Source: CAD feature listing. Evaluate the final solid. Frame: model axes, mm. A direction names the side the tool comes from. Round coordinates to 2 decimals unless told otherwise and drop trailing zeros. Order: outer loops, then holes, each group sorted by start corner. A loop starts at its lowest first (then second) coordinate and runs counter-clockwise, first axis right, second up. Notation, with made-up numbers: (59, 77) - (95, 77) arc R26 ccw to (95, 108) - close; hole circle Ø4 at (-4.5, 69). An arc over 180 degrees is marked (long way). Put each result on its own line as item: value. Start each with the question number.
1) Mould query, pull axis Z, two halves, no side actions, for faces 4 (the face through (-13, 16, 70)), 5 (the face through (3, 0, 100)), 6 (the face through (0, -2, 0)), 7 (the face through (-5, 5, 80)). Classes: +Z half, -Z half, draft (parallel to the pull), parting line (faces both ways), or undercut.
2) Access query for faces 1 (the face through (-13, 16, 50)), 2 (the face through (-14.985, 0.66, 23.269)), 3 (the face through (-1, 0, 115)). Directions: +Z, -Z, +X, -X, +Y, -Y. A direction counts if a zero-diameter tool reaches every point of the face in a straight line with its end or side. Return the directions, or none.
3) Line query: probe 1 along Z at (x, y) = (13, -17.5); probe 2 along Z at (x, y) = (5, 2); probe 3 along Z at (x, y) = (-9, -13.5). Output: solid intervals per line, ascending. Write a range as [from, to].
4) Section B-B on y = -17. Output: boundary loops of the cut face in (x, z), then the cut area to 3 significant figures.
5) Contact query for flat-ended pins moving along their axis: P1, Ø2, axis at y = 5.5, z = 19, coming from the -X side; P2, Ø0.6, axis at x = 4, y = 1, coming from the +Z side; P3, Ø4, axis at x = 7.5, y = -1, coming from the -Z side. Output: stop coordinate, or through.
6) Section A-A on z = 57. Output: boundary loops of the cut face in (x, y).
```python
from build123d import *

# Parameters (mm, degrees)
SKETCH1_R           = 15
BOSS_EXTRUDE1_DEPTH = 40
SKETCH2_W           = 42
SKETCH2_H           = 42
BOSS_EXTRUDE4_DEPTH = 10
SKETCH3_R           = 20
BOSS_EXTRUDE5_DEPTH = 20
SKETCH4_W           = 42
SKETCH4_H           = 42
BOSS_EXTRUDE6_DEPTH = 10
SKETCH5_R           = 5
BOSS_EXTRUDE7_DEPTH = 35
FILLET3_R           = 7
SKETCH6_R           = 1.25
BOSS_EXTRUDE8_DEPTH = 5
FILLET5_R           = 0.3
SKETCH7_W           = 4
SKETCH7_H           = 6
CUT_EXTRUDE1_DEPTH  = 30


with BuildPart() as part:
    # Sketch1 → Boss-Extrude1 (new body)
    with BuildSketch(Plane.XY):
        Circle(SKETCH1_R)
    extrude(amount=BOSS_EXTRUDE1_DEPTH)

    # Sketch2 → Boss-Extrude4 (add)
    with BuildSketch(Plane.XY.offset(40)):
        Rectangle(SKETCH2_W, SKETCH2_H)
    extrude(amount=BOSS_EXTRUDE4_DEPTH)

    # Sketch3 → Boss-Extrude5 (add)
    with BuildSketch(Plane.XY.offset(50)):
        Circle(SKETCH3_R)
    extrude(amount=BOSS_EXTRUDE5_DEPTH)

    # Sketch4 → Boss-Extrude6 (add)
    with BuildSketch(Plane.XY.offset(70)):
        Rectangle(SKETCH4_W, SKETCH4_H)
    extrude(amount=BOSS_EXTRUDE6_DEPTH)

    # Sketch5 → Boss-Extrude7 (add)
    with BuildSketch(Plane.XY.offset(80)):
        Circle(SKETCH5_R)
    extrude(amount=BOSS_EXTRUDE7_DEPTH)

    # Fillet3
    fillet3_edges = [part.edges().sort_by_distance(p)[0] for p in [
        (-15, 0, 0),
    ]]
    fillet(fillet3_edges, radius=FILLET3_R)

    # Sketch6 → Boss-Extrude8 (add)
    with BuildSketch(Plane(origin=(0, 0, 0), x_dir=(-1, 0, 0), z_dir=(0, 0, -1))):
        with Locations(Location((0, 0, 0), (0, 0, 180))):
            Circle(SKETCH6_R)
    extrude(amount=BOSS_EXTRUDE8_DEPTH)

    # Fillet5
    fillet5_edges = [part.edges().sort_by_distance(p)[0] for p in [
        (-1.25, 0, -5),
    ]]
    fillet(fillet5_edges, radius=FILLET5_R)

    # Sketch7 → Cut-Extrude1 (cut)
    with BuildSketch(Plane.XY.offset(115)):
        with Locations((5, 0)):
            Rectangle(SKETCH7_W, SKETCH7_H)
    extrude(amount=-CUT_EXTRUDE1_DEPTH, mode=Mode.SUBTRACT)


solid = part.part
```
Answer sheet:
1. face 4: undercut
1. face 5: draft
1. face 6: -Z half
1. face 7: +Z half
2. face 1: none
2. face 2: -Z
2. face 3: +Z, +X, -X, +Y, -Y
3. probe 1: [40, 50], [70, 80]
3. probe 2: [0, 80]
3. probe 3: [40, 80]
4. outline: (-21, 40) - (21, 40) - (21, 50) - (10.54, 50) - (10.54, 70) - (21, 70) - (21, 80) - (-21, 80) - (-21, 70) - (-10.54, 70) - (-10.54, 50) - (-21, 50) - close
4. area: 1,260 mm^2
5. P1: x = -14.31
5. P2: z = 85
5. P3: z = 0
6. outline: circle Ø40 at (0, 0)
